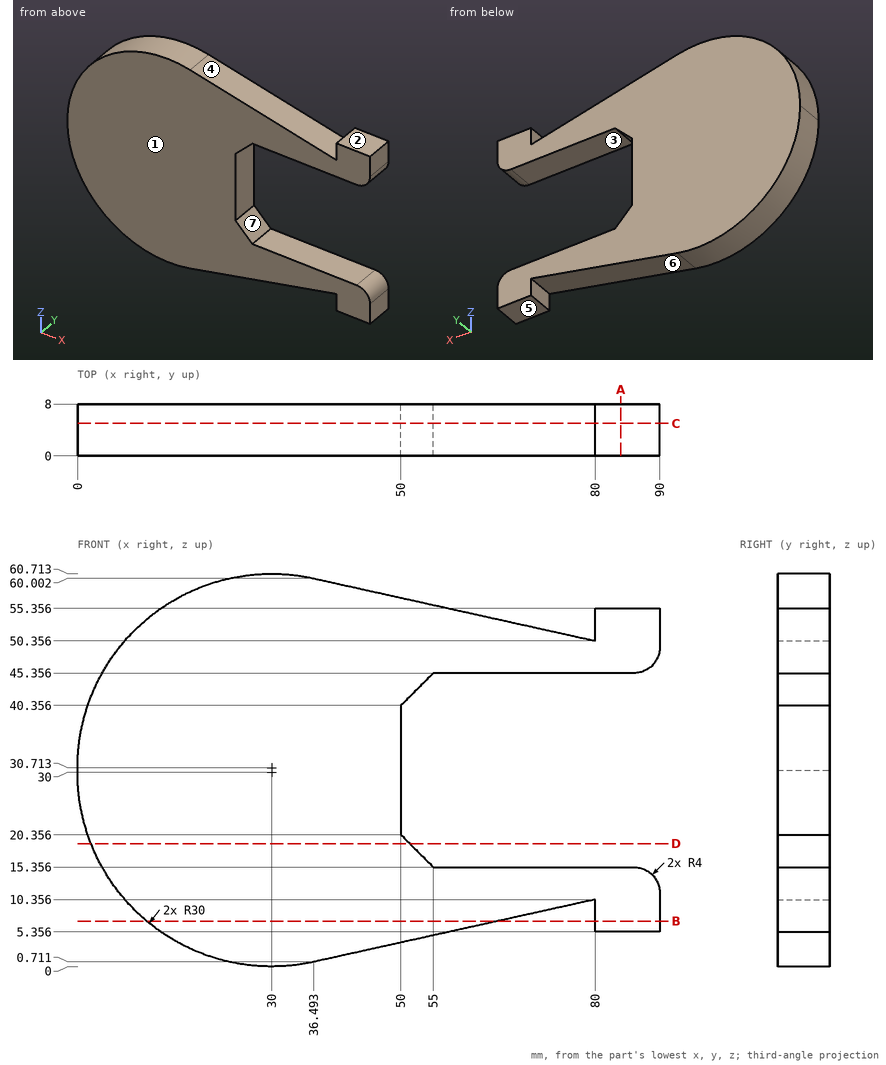
Design review of the part shown in the three views and the two pictorial views. Dimensions are in mm from the part's minimum x, y and z. A direction names the side the tool comes from. Round coordinates to 2 decimals unless told otherwise and drop trailing zeros. Loops run counter-clockwise (first coordinate to the right, second up) from the corner with the lowest first, then second, coordinate; pieces in that order, holes last.
1) Tool access review of the marked faces 1, 2, 3 and 4: name each direction out of +Z, -Z, +X, -X, +Y, -Y from which nothing blocks a thin tool from reaching the whole face with its end or side.
Values follow:
face 1: +Z, -Z, +X, -X, -Y
face 2: +Z, +X, +Y, -Y
face 3: +X, +Y, -Y
face 4: +Z, +Y, -Y
2) Consider section A-A on x = 84. State the section outline as (y, z) points.
Values follow:
outline: (0, 5.36) - (8, 5.36) - (8, 15.36) - (0, 15.36) - close; (0, 45.36) - (8, 45.36) - (8, 55.36) - (0, 55.36) - close
3) Wall thickness on line 1 along Z through (x, y) = (82, 2); line 2 along Z through (x, y) = (54.5, 2.75) (1 decimal); line 3 along X through (y, z) = (0.75, 31.5): over which ranges is each line inside the solid? List them lowest first.
Values follow:
line 1: z = 5.36 to 15.36, 45.36 to 55.36
line 2: z = 4.7 to 15.9, 44.9 to 56
line 3: x = 0.01 to 50
4) Clearance check with flat-ended pins moving along their axes: P1, Ø2.5, axis at y = 2.5, z = 7, coming from the -X side; P2, Ø4, axis at x = 73, y = 3, coming from the +Z side; P3, Ø4, axis at y = 7, z = 11, coming from the -X side. State where each tip first meets the part, or that it passes through.
Values follow:
P1: stops at x = 9.34
P2: stops at z = 52.35
P3: stops at x = 5.28
5) Consider section B-B on z = 7. State the section outline as (x, y) points.
Values follow:
outline: (10.74, 0) - (64.86, 0) - (64.86, 8) - (10.74, 8) - close; (80, 0) - (90, 0) - (90, 8) - (80, 8) - close
6) The part is to be moulded in two halves that separate along X. For the marked faces 5, 6 and 7, say which applies: pulls with the +X half, pulls with the -X half, needs draft (parallel to the pull), parting line crosses it, or undercut.
Values follow:
face 5: needs draft
face 6: undercut
face 7: pulls with the +X half
7) Consider section C-C on y = 5. State the section outline as (x, z) points.
Values follow:
outline: (0, 30.36) arc R30 ccw to (36.49, 0.71) - (80, 10.36) - (80, 5.36) - (90, 5.36) - (90, 11.36) arc R4 ccw to (86, 15.36) - (55, 15.36) - (50, 20.36) - (50, 40.36) - (55, 45.36) - (86, 45.36) arc R4 ccw to (90, 49.36) - (90, 55.36) - (80, 55.36) - (80, 50.36) - (36.49, 60) arc R30 ccw to start
8) Consider section D-D on z = 19. State the section outline as (x, y) points, then the cut area to 3 significant figures.
Values follow:
outline: (2.09, 0) - (51.36, 0) - (51.36, 8) - (2.09, 8) - close
area: 394 mm2
